Autodesk Inventor part; units mm, degrees
ref_plane "YZ Plane" through (0, 0, 0) normal (1, 0, 0) x (0, 1, 0)
ref_plane "XZ Plane" through (0, 0, 0) normal (0, 1, 0) x (-1, 0, 0)
ref_plane "XY Plane" through (0, 0, 0) normal (0, 0, 1) x (1, 0, 0)
sketch "Sketch1" plane through (0, 0, 0) normal (1, 0, 0) x (0, 1, 0)
  circle A0 centre (0, 0) radius 20
  dimension "d0" = 40
extrude "Extrusion1" add sketch "Sketch1" along normal blind 17.5
sketch "Sketch2" plane through (17.5, 0, 0) normal (1, 0, 0) x (0, 0, -1)
  circle A0 centre (0, 0) radius 3
  circle A1 centre (0, 0) radius 1.5
  dimension "d3" = 6
  dimension "d4" = 3
extrude "Extrusion2" add sketch "Sketch2" against normal blind 22
sketch "Sketch3" plane through (0, 0, 0) normal (-1, 0, 0) x (0, 0, 1)
  circle A0 centre (0, 0) radius 1.5
  circle A1 centre (0, 0) radius 1.5
extrude "Extrusion3" cut sketch "Sketch3" against normal blind 50
sketch "Sketch4" plane through (17.5, 0, 0) normal (1, 0, 0) x (0, 0, -1)
  circle A0 centre (0, 0) radius 12.5
  dimension "d9" = 25
extrude "Extrusion4" cut sketch "Sketch4" against normal blind 8
sketch "Sketch5" plane through (0, 0, 0) normal (-1, 0, 0) x (0, 0, 1)
  circle A0 centre (0, 0) radius 12.5
  circle A1 centre (0, 0) radius 3
  dimension "d12" = 25
extrude "Extrusion5" cut sketch "Sketch5" against normal blind 8
properties part number "Back Wheel" material "PC/ABS Plastic"
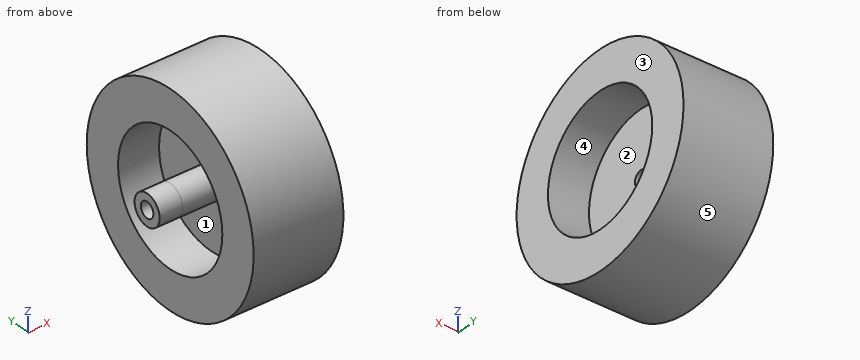
Geometry: final body of the model. Coordinates: model frame, mm. Face numbers are marked on the shaded views. A direction names the side the tool comes from. Coordinates: 2 decimals unless noted, no trailing zeros. Loops run counter-clockwise (first coordinate to the right, second up) from the corner with the lowest first, then second, coordinate; pieces in that order, holes last. Notation, with made-up numbers: M 3.25,61 L 16.25,61 A21 cw 16.25,71 Z; hole C -40,14 d6. An arc over 180 degrees is marked long. Put each result on its own line as item: value.
(1) Material intervals for probe 1 along Y at (x, z) = (6.25, -2); probe 2 along X at (y, z) = (8.5, -11.5); probe 3 along Y at (x, z) = (14.75, 11.5), sorted ascending.
Answer sheet:
probe 1: y = -19.9 to -12.34, -2.24 to 2.24, 12.34 to 19.9
probe 2: x = 0 to 17.5
probe 3: y = -16.36 to -4.9, 4.9 to 16.36
(2) Cut plane B-B on x = 4.5. Return the cut outline in (y, z), then the cut area to 3 significant figures.
Answer sheet:
outline: C 0,0 d40; C 0,0 d6; hole C 0,0 d25; hole C 0,0 d3
area: 787 mm^2
(3) Cut plane D-D on x = -1.5. Return the cut outline in (y, z).
Answer sheet:
outline: C 0,0 d6; hole C 0,0 d3
(4) Access query for the marked faces 1 and 2. Directions: +Z, -Z, +X, -X, +Y, -Y. A direction counts if a zero-diameter tool reaches every point of the face in a straight line with its end or side. Return the directions, or none.
Answer sheet:
face 1: -X
face 2: +X
(5) First-contact query: pin 1 (5 mm diameter, centred on y = 0, z = 0, fed in from +X); pin 2 (2 mm diameter, centred on x = 7.5, z = 4, fed in from +Y); pin 3 (1 mm diameter, centred on x = -1.5, y = 5.5, fed in from -Z); pin 4 (1.5 mm diameter, centred on x = 0.5, z = 15, fed in from -Y). Flat tips, straight axial feed; report the tip coordinate or a pass-through.
Answer sheet:
pin 1: stops at x = 9.5
pin 2: stops at y = 19.77
pin 3: passes through
pin 4: stops at y = -14.03
(6) Draft query along Y for the marked faces 3, 4 and 5. Return one class per face: pulls with the +Y half, pulls with the -Y half, needs draft (parallel to the pull), parting line crosses it, or undercut.
Answer sheet:
face 3: needs draft
face 4: undercut
face 5: parting line crosses it
(7) Cut plane A-A on y = 0. Return the cut outline in (x, z).
Answer sheet:
outline: M -4.5,-3 L 8,-3 L 8,-12.5 L 0,-12.5 L 0,-20 L 17.5,-20 L 17.5,-12.5 L 9.5,-12.5 L 9.5,-1.5 L -4.5,-1.5 Z; M -4.5,1.5 L 9.5,1.5 L 9.5,12.5 L 17.5,12.5 L 17.5,20 L 0,20 L 0,12.5 L 8,12.5 L 8,3 L -4.5,3 Z
